Geometry check sheet. Reference: the model listing, model coordinates, mm. A direction names the side the tool comes from. Round coordinates to 2 decimals unless told otherwise and drop trailing zeros. Write each loop counter-clockwise with the first axis right and the second up, starting at its lowest first coordinate (ties: lowest second). Pieces come first, ordered by that corner, then holes. Notation, with made-up numbers: M -39,-29 L -12,-29 A18 ccw -12,-25 Z; hole C 70.5,33 d2. An arc over 180 degrees is marked long. Put each result on its own line as item: value. Start each with the question number.
(1) Section check A-A on y = 95.5. Record the cut outline in (x, z), then the cut area to 3 significant figures.
(2) Gauge pin test, flat ends, axial feed: pin 1 (10 mm diameter, centred on y = 118, z = -55.5, fed in from -X); pin 2 (2.5 mm diameter, centred on x = -103.5, y = 43.5, fed in from +Z); pin 3 (0.8 mm diameter, centred on x = -100.5, y = 52, fed in from -Z). Record the tip position at first contact, or that the pin passes through.
(3) Tool access check on faces 1 (the flat face through (-52, 180, -85)), 2 (the flat face through (-10, 120, -55.811)), 3 (the flat face through (-103, 60.366, -48)), 4 (the flat face through (-103, 45, -69.132)), 5 (the cylindrical face through (-92.6, 65.78, -59.08)). Record the directions out of +Z, -Z, +X, -X, +Y, -Y that give a thin tool (end or side, any length) a straight path to the whole face; none if there is none.
(4) Material ranges on probe 1 along Z at (x, y) = (-35.5, -42); probe 2 along Z at (x, y) = (-46, 25); probe 3 along Z at (x, y) = (-43, 128), recorded low to high.
(5) Section check D-D on x = -36. Record the cut outline in (y, z), then the cut area to 3 significant figures.
(6) Section check C-C on z = -32. Record the cut outline in (x, y), then the cut area to 3 significant figures.
(7) Mould release check, pull along Y, two halves, no side actions. Record for faces 6 (the flat face through (0, 71, -56)), 7 (the flat face through (-85, 65, -57)), 8 (the flat face through (-49.9, 7.5, -6.6)): pulls with the +Y half, pulls with the -Y half, needs draft (parallel to the pull), parting line crosses it, or undercut.
(8) Section check B-B on x = -95.5. Record the cut outline in (y, z).
from build123d import *

# Parameters (mm, degrees)
SKETCH1_W           = 100
SKETCH1_H           = 100
BOSS_EXTRUDE1_DEPTH = 180
SKETCH2_R           = 34.257790197
BOSS_EXTRUDE2_DEPTH = 350
SKETCH3_W           = 152.006357392
SKETCH3_H           = 282.452416457
CUT_EXTRUDE2_DEPTH  = 400
CUT_EXTRUDE3_DEPTH  = 400
CUT_EXTRUDE4_DEPTH  = 400
CUT_EXTRUDE5_DEPTH  = 400
SKETCH7_W           = 160.159381639
SKETCH7_H           = 147.362276113
CUT_EXTRUDE6_DEPTH  = 400
SKETCH8_W           = 147.310744502
SKETCH8_H           = 162.038906966
CUT_EXTRUDE7_DEPTH  = 400
SKETCH9_R           = 31.847293423
CUT_EXTRUDE8_DEPTH  = 400
SKETCH10_W          = 140.220962397
SKETCH10_H          = 212.033531124
CUT_EXTRUDE9_DEPTH  = 400
SKETCH11_R          = 13.603137886
CUT_EXTRUDE11_DEPTH = 15
SKETCH12_R          = 12.495422516
BOSS_EXTRUDE3_DEPTH = 15
SKETCH13_R          = 1.594865099
BOSS_EXTRUDE4_DEPTH = 4
SKETCH14_W          = 100.74862993
SKETCH14_H          = 110.555003588
CUT_EXTRUDE13_DEPTH = 400
BOSS_EXTRUDE5_DEPTH = 1
SKETCH16_W          = 42.108585165
SKETCH16_H          = 30.458347221
BOSS_EXTRUDE6_DEPTH = 5
SKETCH17_W          = 18.669530869
SKETCH17_H          = 22.4027039
BOSS_EXTRUDE7_DEPTH = 1
SKETCH18_W          = 4.907623399
SKETCH18_H          = 5.170746831
SKETCH18_W_2        = 3.981473695
SKETCH18_H_2        = 5.451349552
BOSS_EXTRUDE8_DEPTH = 1
BOSS_EXTRUDE9_DEPTH = 1


with BuildPart() as part:
    # Sketch1 → Boss-Extrude1 (new body)
    with BuildSketch(Plane(origin=(0, 0, 0), x_dir=(1, 0, 0), z_dir=(0, 1, 0))):
        with Locations((-50, 50)):
            Rectangle(SKETCH1_W, SKETCH1_H)
    extrude(amount=BOSS_EXTRUDE1_DEPTH)

    # Sketch2 → Boss-Extrude2 (add, symmetric)
    with BuildSketch(Plane(origin=(0, 180, 0), x_dir=(1, 0, 0), z_dir=(0, 1, 0))):
        with Locations(Location((-51.377291833, 49.076536384, 0), (0, 0, 270))):
            Circle(SKETCH2_R)
    extrude(amount=BOSS_EXTRUDE2_DEPTH, both=True)

    # Sketch3 → Cut-Extrude2 (cut)
    with BuildSketch(Plane(origin=(0, 0, 0), x_dir=(0, 0, -1), z_dir=(1, 0, 0))):
        with Locations((57.419900112, 502.274302507)):
            Rectangle(SKETCH3_W, SKETCH3_H)
    extrude(amount=-CUT_EXTRUDE2_DEPTH, mode=Mode.SUBTRACT)

    # Sketch4 → Cut-Extrude3 (cut)
    with BuildSketch(Plane(origin=(0, 0, 0), x_dir=(0, 0, -1), z_dir=(1, 0, 0))):
        Polygon((12.981970869, 0), (-8.994244796, 25.828096003), (-18.564506014, -15.259465835), align=None)
        Polygon((85.072517936, -1.448103984), (109.237639161, 19.113145112), (115.920034239, -3.267382694), align=None)
        Polygon((12.981970869, 180), (-8.994244796, 148.537596011), (-15.418178585, 193.219274892), align=None)
        Polygon((85.072517936, 181.854312784), (103.841225373, 159.795920888), (106.132549481, 198.647393934), align=None)
    extrude(amount=-CUT_EXTRUDE3_DEPTH, mode=Mode.SUBTRACT)

    # Sketch5 → Cut-Extrude4 (cut)
    with BuildSketch(Plane.XY):
        Polygon((-85.623287335, 0), (-106.370377984, 21.426392531), (-122.288861874, 3.209259887), (-93.526345261, -19.884701759), align=None)
        Polygon((-15.694988751, 0), (0, 15.257385304), (12.122677088, 15.257385304), (10.563067769, -19.884701759), align=None)
        Polygon((-87.166490339, 180.248071029), (-106.370377984, 151.29108453), (-117.705469457, 200.501115102), align=None)
        Polygon((-15.694988751, 180.248071029), (7.833767065, 153.279557508), (0, 193.941208308), align=None)
    extrude(amount=-CUT_EXTRUDE4_DEPTH, mode=Mode.SUBTRACT)

    # Sketch6 → Cut-Extrude5 (cut)
    with BuildSketch(Plane(origin=(0, 180, 0), x_dir=(1, 0, 0), z_dir=(0, 1, 0))):
        Polygon((-112.386997555, 28.400400964), (-64.261264503, -10.212759359), (-84.406366528, -15.51192827), (-124.649689542, -15.51192827), align=None)
        Polygon((-97.065537028, 135.861756084), (-119.37552445, 77.792688888), (-118.043343626, 64.347606737), (-66.428694172, 110.575168787), align=None)
        Polygon((-24.69640689, -21.815840769), (11.092108798, -8.97361337), (17.428316417, 32.393768119), (-38.531576846, -11.139157378), align=None)
        Polygon((-17.445484601, 140.804394854), (35.417473102, 107.262520599), (9.305452855, 72.996438725), (-31.724385352, 103.625272537), align=None)
    extrude(amount=-CUT_EXTRUDE5_DEPTH, mode=Mode.SUBTRACT)

    # Sketch7 → Cut-Extrude6 (cut)
    with BuildSketch(Plane.XY):
        with Locations((-66.123258915, -136.36252694)):
            Rectangle(SKETCH7_W, SKETCH7_H)
    extrude(amount=-CUT_EXTRUDE6_DEPTH, mode=Mode.SUBTRACT)

    # Sketch8 → Cut-Extrude7 (cut)
    with BuildSketch(Plane.XY):
        with Locations((-53.541153336, 332.448287589)):
            Rectangle(SKETCH8_W, SKETCH8_H)
    extrude(amount=-CUT_EXTRUDE7_DEPTH, mode=Mode.SUBTRACT)

    # Sketch9 → Cut-Extrude8 (cut)
    with BuildSketch(Plane(origin=(0, 251.428834106, 0), x_dir=(1, 0, 0), z_dir=(0, 1, 0))):
        with Locations(Location((-50.808993157, 49.032036374, 0), (0, 0, 270))):
            Circle(SKETCH9_R)
    extrude(amount=-CUT_EXTRUDE8_DEPTH, mode=Mode.SUBTRACT)

    # Sketch10 → Cut-Extrude9 (cut)
    with BuildSketch(Plane.ZY.offset(100)):
        with Locations((14.299084536, 180.100625535)):
            Rectangle(SKETCH10_W, SKETCH10_H)
    extrude(amount=-CUT_EXTRUDE9_DEPTH, mode=Mode.SUBTRACT)

    # Sketch11 → Cut-Extrude11 (cut)
    with BuildSketch(Plane.ZY.offset(100)):
        with Locations((-50.413251954, 76.264646142)):
            Circle(SKETCH11_R)
    extrude(amount=-CUT_EXTRUDE11_DEPTH, mode=Mode.SUBTRACT)

    # Sketch12 → Boss-Extrude3 (add)
    with BuildSketch(Plane.ZY.offset(85)):
        with Locations(Location((-50.658800768, 76.222522328, 0), (0, 0, 114.353089558))):
            Circle(SKETCH12_R)
    extrude(amount=BOSS_EXTRUDE3_DEPTH)

    # Sketch13 → Boss-Extrude4 (add)
    with BuildSketch(Plane(origin=(-85, 0, 0), x_dir=(0, 0, -1), z_dir=(1, 0, 0))):
        with Locations(Location((49.945205578, 75.944780088, 0), (0, 0, 180))):
            Circle(SKETCH13_R)
    extrude(amount=BOSS_EXTRUDE4_DEPTH)

    # Sketch14 → Cut-Extrude13 (cut)
    with BuildSketch(Plane.ZY.offset(100)):
        with Locations((-65.350029467, 250.603414818)):
            Rectangle(SKETCH14_W, SKETCH14_H)
    extrude(amount=-CUT_EXTRUDE13_DEPTH, mode=Mode.SUBTRACT)

    # Sketch15 → Boss-Extrude5 (add)
    with BuildSketch(Plane.ZY.offset(100)):
        Polygon((-18.461827727, 14.847435435), (-80.507743362, 14.847435435), (-80.507743362, 160.896793159), (-55.811396663, 160.896793159), (-55.811396663, 74.083859973), (-18.461827727, 74.083859973), align=None)
    extrude(amount=BOSS_EXTRUDE5_DEPTH)

    # Sketch16 → Boss-Extrude6 (add)
    with BuildSketch(Plane.ZY.offset(101)):
        with Locations((-48.07732297, 45.136437142)):
            Rectangle(SKETCH16_W, SKETCH16_H)
    extrude(amount=BOSS_EXTRUDE6_DEPTH)

    # Sketch17 → Boss-Extrude7 (add)
    with BuildSketch(Plane.ZY.offset(101)):
        with Locations((-67.04663872, 130.409241603)):
            Rectangle(SKETCH17_W, SKETCH17_H)
    extrude(amount=BOSS_EXTRUDE7_DEPTH)

    # Sketch18 → Boss-Extrude8 (add)
    with BuildSketch(Plane.ZY.offset(102)):
        with Locations((-71.625108618, 130.213401885)):
            Rectangle(SKETCH18_W, SKETCH18_H)
        with Locations((-62.297675883, 129.867186512)):
            Rectangle(SKETCH18_W_2, SKETCH18_H_2)
    extrude(amount=BOSS_EXTRUDE8_DEPTH)

    # Sketch19 → Boss-Extrude9 (add)
    with BuildSketch(Plane.ZY.offset(102)):
        Polygon((-66.976455081, 134.868836652), (-73.7929295, 134.868836652), (-73.7929295, 134.108269479), (-74.571872104, 134.108269479), (-74.571872104, 140.512729543), (-73.7929295, 140.512729543), (-72.165965418, 140.512729543), (-72.233411796, 137.421948277), (-71.48458153, 137.421948277), (-71.410861795, 140.512729543), (-69.158339735, 140.504865112), (-69.158339735, 137.421948277), (-68.22174926, 137.421948277), (-68.22174926, 140.567922793), (-65.426885805, 140.567922793), (-65.515241968, 137.446210948), (-64.714122339, 137.446210948), (-64.714122339, 140.567922793), (-62.410871788, 140.567922793), (-62.410871788, 137.210126003), (-61.403493639, 137.210126003), (-61.403493639, 140.631129361), (-58.889974549, 140.631129361), (-58.889974549, 136.595539338), (-59.698319644, 136.595539338), (-59.698319644, 139.99489006), (-60.695848378, 139.984078324), (-60.695848378, 136.667717235), (-63.090112056, 136.667717235), (-63.090112056, 139.979723883), (-64.00479018, 139.979723883), (-64.00479018, 136.667717235), (-66.334605538, 136.667717235), (-66.334605538, 139.902697072), (-67.48995239, 139.902697072), (-67.48995239, 136.667717235), (-70.008746759, 136.667717235), (-70.008746759, 139.902697072), (-70.709698815, 139.902697072), (-70.783897489, 136.693128041), (-72.921241048, 136.693128041), (-72.921241048, 139.545601992), (-73.7929295, 139.545601992), (-73.7929295, 135.423339258), (-66.976455081, 135.49721976), align=None)
    extrude(amount=BOSS_EXTRUDE9_DEPTH)


solid = part.part
Answers follow:
1. outline: M -101,-80.51 L -100,-80.51 L -78.24,-100 L -26.87,-100 L 0,-79.94 L 0,-55.81 L -19.69,-55.81 A31.85 cw -81.93,-55.81 L -101,-55.81 Z
1. area: 2,800 mm^2
2. pin 1: stops at x = -102
2. pin 2: stops at z = -27.02
2. pin 3: stops at z = -80.51
3. face 1: -Z, +Y
3. face 2: +Z, +X, +Y
3. face 3: +Z, -Z, -X
3. face 4: -Z, -X, -Y
3. face 5: none
4. probe 1: z = -79.43 to -76.96, -21.11 to -18.72
4. probe 2: z = -100 to -80.51, -17.55 to 0
4. probe 3: z = -100 to -79.91
5. outline: M -62.68,-79.69 L 0,-79.69 L 0,-86.77 L 11.25,-100 L 164.31,-100 L 180,-86.65 L 180,-79.69 L 195.33,-79.69 L 195.33,-77.23 L -62.68,-77.23 Z; M -62.68,-20.84 L 74.08,-20.84 L 74.08,0 L 15.26,0 L 0,-12.98 L 0,-18.46 L -62.68,-18.46 Z
5. area: 5,710 mm^2
6. outline: M -106,29.91 L -101,29.91 L -101,14.85 L -100,14.85 L -85.62,0 L -81.08,0 L -81.08,-62.68 L -77.72,-62.68 L -77.72,74.08 L -101,74.08 L -101,60.37 L -106,60.37 Z; M -23.9,-62.68 L -21.68,-62.68 L -21.68,0 L -15.69,0 L 0,15.26 L 0,74.08 L -23.9,74.08 Z
6. area: 3,760 mm^2
7. face 6: needs draft
7. face 7: undercut
7. face 8: pulls with the -Y half
8. outline: M 10.2,-84.54 L 167.68,-84.54 L 167.68,-55.81 L 88.75,-55.81 A13.6 cw long 74.08,-36.99 L 74.08,-14.85 L 10.2,-14.85 Z; C 76.22,-50.66 d24.99
